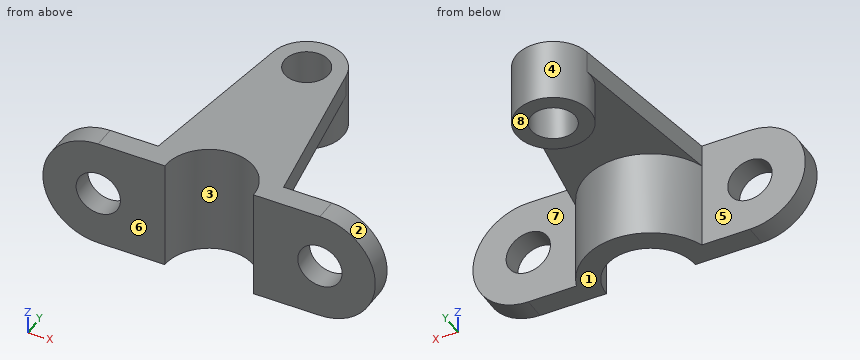
from build123d import *

# Parameters (mm, degrees)
BOSS_EXTRUDE1_DEPTH = 30
BOSS_EXTRUDE2_DEPTH = 12
SKETCH4_R           = 20
BOSS_EXTRUDE3_DEPTH = 34
SKETCH4_3_R         = 12
CUT_EXTRUDE1_DEPTH  = 34
BOSS_EXTRUDE4_DEPTH = 12
SKETCH5_R           = 12
CUT_EXTRUDE2_DEPTH  = 144.291935896


with BuildPart() as part:
    # Sketch2 → Boss-Extrude1 (new, symmetric)
    with BuildSketch(Plane.XY):
        with BuildLine():
            Line((-36, 0), (-24, 0))
            ThreePointArc((-24, 0), (0, 24), (24, 0))
            Line((24, 0), (36, 0))
            ThreePointArc((36, 0), (0, 36), (-36, 0))
        make_face()
    extrude(amount=BOSS_EXTRUDE1_DEPTH, both=True)

    # Sketch3 → Boss-Extrude2 (add)
    with BuildSketch(Plane(origin=(0, 0, 0), x_dir=(1, 0, 0), z_dir=(0, 1, 0))):
        with BuildLine():
            Line((36, 30), (60, 30))
            ThreePointArc((60, 30), (90, 0), (60, -30))
            Line((60, -30), (36, -30))
            Line((36, -30), (30, -30))
            Line((30, -30), (30, 30))
            Line((30, 30), (36, 30))
        make_face()
        with BuildLine():
            Line((-30, 30), (-36, 30))
            Line((-36, 30), (-60, 30))
            ThreePointArc((-60, 30), (-90, 0), (-60, -30))
            Line((-60, -30), (-36, -30))
            Line((-36, -30), (-30, -30))
            Line((-30, -30), (-30, 30))
        make_face()
    extrude(amount=BOSS_EXTRUDE2_DEPTH)



with BuildPart() as body_2:
    # Sketch4 → Boss-Extrude3 (new body)
    with BuildSketch(Plane.XY.offset(30)):
        with Locations((0, 99.389845389)):
            Circle(SKETCH4_R)
    extrude(amount=-BOSS_EXTRUDE3_DEPTH)

    # Sketch4_3 → Cut-Extrude1 (cut)
    with BuildSketch(Plane.XY.offset(30)):
        with Locations((0, 99.389845389)):
            Circle(SKETCH4_3_R)
    extrude(amount=-CUT_EXTRUDE1_DEPTH, mode=Mode.SUBTRACT)


with BuildPart() as part_1:
    add(part.part)

    add(body_2.part)  # Boss-Extrude4 merges body 2
    # Sketch4_4 → Boss-Extrude4 (add)
    with BuildSketch(Plane.XY.offset(30)):
        with BuildLine():
            Line((0, 79.389845389), (0, 36))
            ThreePointArc((0, 36), (20.784609691, 29.393876913), (33.941125497, 12))
            Line((33.941125497, 12), (19.75877981, 102.486718075))
            ThreePointArc((19.75877981, 102.486718075), (19.93960376, 100.942971882), (20, 99.389845389))
            ThreePointArc((20, 99.389845389), (14.142135624, 85.247709765), (0, 79.389845389))
        make_face()
        with BuildLine():
            ThreePointArc((-33.941125497, 12), (-20.784609691, 29.393876913), (0, 36))
            Line((0, 36), (0, 79.389845389))
            ThreePointArc((0, 79.389845389), (-15.197655308, 86.388642631), (-19.75877981, 102.486718075))
            Line((-19.75877981, 102.486718075), (-33.941125497, 12))
        make_face()
    extrude(amount=-BOSS_EXTRUDE4_DEPTH)

    # Sketch5 → Cut-Extrude2 (cut, through all)
    with BuildSketch(Plane(origin=(0, 12, 0), x_dir=(1, 0, 0), z_dir=(0, 1, 0))):
        with Locations(Location((-60, 0, 0), (0, 0, 270))):
            Circle(SKETCH5_R)
    cut_extrude2 = extrude(amount=-CUT_EXTRUDE2_DEPTH, mode=Mode.SUBTRACT)

    # Mirror1: Cut-Extrude2 across plane
    add(cut_extrude2.mirror(Plane(origin=(0, 0, 0), x_dir=(0, 0, 1), z_dir=(1, 0, 0))), mode=Mode.SUBTRACT)


solid = part_1.part
The listing builds one solid part. Answer for the finished solid, in the listing's coordinates (mm). Face numbers are marked on the shaded views. A direction names the side the tool comes from. Give positions to 0.01 mm unless a question says otherwise; leave off trailing zeros. Loops run counter-clockwise (first coordinate to the right, second up) from the corner with the lowest first, then second, coordinate; pieces in that order, holes last.
Item 1: A cutting plane is placed at A-A (z = 0). Give the vertices of the cut face in (x, y).
Derived:
outline: (-90, 0) - (-72, 0) - (-72, 12) - (-90, 12) - close; (-48, 0) - (-24, 0) arc R24 cw to (24, 0) - (48, 0) - (48, 12) - (33.94, 12) arc R36 ccw to (-33.94, 12) - (-48, 12) - close; circle Ø40 at (0, 99.39); (72, 0) - (90, 0) - (90, 12) - (72, 12) - close; hole circle Ø24 at (0, 99.39)
Item 2: Determine the mould class of the marked faces 1, 2 and 3 for opening direction X: +X half, -X half, draft (parallel to the pull), parting line (faces both ways), or undercut.
Derived:
face 1: draft
face 2: +X half
face 3: undercut
Item 3: A cutting plane is placed at B-B (x = 53). Give the vertices of the cut face in (y, z), then the cut area to 3 significant figures.
Derived:
outline: (0, -30) - (12, -30) - (12, -9.75) - (0, -9.75) - close; (0, 9.75) - (12, 9.75) - (12, 30) - (0, 30) - close
area: 486 mm2
Item 4: A cutting plane is placed at D-D (z = -18). Give the vertices of the cut face in (x, y).
Derived:
outline: (-84, 0) - (-24, 0) arc R24 cw to (24, 0) - (84, 0) - (84, 12) - (33.94, 12) arc R36 ccw to (-33.94, 12) - (-84, 12) - close
Item 5: A tool of negligible diameter and unlimited length cuts with its end or side. For the marked faces 4, 5, 6, 7 and 8, from which of +Z, -Z, +X, -X, +Y, -Y can it reach the whole face along a straight path? Write none if from no direction.
Derived:
face 4: -Z
face 5: +Z, -Z, -X, +Y
face 6: +Z, -Z, +X, -X, -Y
face 7: +Z, -Z, +X, +Y
face 8: -Z, +X, -X, +Y
Item 6: Each of these flat-tipped pins is pushed along its axis until it touches: pin 1 Ø3 at (x, z) = (57, -20.5) entering from +Y; pin 2 Ø21.5 at (x, y) = (0, 99.39) entering from -Z (3 decimals); pin 3 Ø2 at (y, z) = (69, 19) entering from -X; pin 4 Ø12 at (y, z) = (95, 2) entering from +X. Where does it stop, or does it pass through?
Derived:
pin 1: stops at y = 12
pin 2: passes through
pin 3: stops at x = -25.16
pin 4: stops at x = 20
Item 7: Find the intervals of material crossed by line 1 along Y through (x, z) = (0, 7); line 2 along X through (y, z) = (8, 0); line 3 along Z through (x, y) = (60, 3), in increasing order.
Derived:
line 1: y = 24 to 36, 79.39 to 87.39, 111.39 to 119.39
line 2: x = -90 to -72, -48 to -22.63, 22.63 to 48, 72 to 90
line 3: z = -30 to -12, 12 to 30
Item 8: A cutting plane is placed at C-C (y = 90). Give the vertices of the cut face in (x, z), then the cut area to 3 significant figures.
Derived:
outline: (-21.72, 18) - (-17.66, 18) - (-17.66, -4) - (-7.47, -4) - (-7.47, 30) - (-21.72, 30) - close; (7.47, -4) - (17.66, -4) - (17.66, 18) - (21.72, 18) - (21.72, 30) - (7.47, 30) - close
area: 790 mm2
